```python
from build123d import *

# Parameters (mm, degrees)
ESQUISSE1_W                     = 85
ESQUISSE1_H                     = 72
BOSS_EXTRU_1_DEPTH              = 5
ESQUISSE3_R                     = 1.5
ENL_V_MAT_EXTRU_5_DEPTH         = 5
ESQUISSE5_R                     = 1.75
ENL_V_MAT_EXTRU_6_DEPTH         = 5
R_P_TITION_LIN_AIRE2_COUNT      = 6
R_P_TITION_LIN_AIRE2_PITCH      = 12
R_P_TITION_LIN_AIRE2_COUNT_DIR2 = 5
R_P_TITION_LIN_AIRE2_PITCH_DIR2 = 12
ESQUISSE6_R                     = 9.852345932
ENL_V_MAT_EXTRU_7_DEPTH         = 5
ESQUISSE8_R                     = 1.5
ENL_V_MAT_EXTRU_8_DEPTH         = 5


with BuildPart() as part:
    # Esquisse1 → Boss.-Extru.1 (new body)
    with BuildSketch(Plane.XY):
        Rectangle(ESQUISSE1_W, ESQUISSE1_H)
    extrude(amount=BOSS_EXTRU_1_DEPTH)

    # Esquisse3 → Enlèv. mat.-Extru.5 (cut)
    with BuildSketch(Plane.ZY.offset(42.5)):
        with Locations((2.5, 0)):
            Circle(ESQUISSE3_R)
    enl_v_mat_extru_5 = extrude(amount=-ENL_V_MAT_EXTRU_5_DEPTH, mode=Mode.SUBTRACT)

    # Symétrie1: Enlèv. mat.-Extru.5 across plane
    add(enl_v_mat_extru_5.mirror(Plane(origin=(0, 0, 0), x_dir=(0, 0, 1), z_dir=(1, 0, 0))), mode=Mode.SUBTRACT)

    # Esquisse5 → Enlèv. mat.-Extru.6 (cut)
    with BuildSketch(Plane.XY):
        with Locations(Location((-31.5, -25, 0), (0, 0, 180))):
            Circle(ESQUISSE5_R)
    enl_v_mat_extru_6 = extrude(amount=ENL_V_MAT_EXTRU_6_DEPTH, mode=Mode.SUBTRACT)

    # Répétition linéaire2: Enl_v. mat.-Extru.6 6 × 5
    with Locations(*[(i * R_P_TITION_LIN_AIRE2_PITCH, j * R_P_TITION_LIN_AIRE2_PITCH_DIR2, 0) for i in range(R_P_TITION_LIN_AIRE2_COUNT) for j in range(R_P_TITION_LIN_AIRE2_COUNT_DIR2) if (i, j) != (0, 0)]):
        add(enl_v_mat_extru_6, mode=Mode.SUBTRACT)

    # Esquisse6 → Enlèv. mat.-Extru.7 (cut)
    with BuildSketch(Plane.XY):
        with Locations(Location((-19.5, -13, 0), (0, 0, 180))):
            Circle(ESQUISSE6_R)
    extrude(amount=ENL_V_MAT_EXTRU_7_DEPTH, mode=Mode.SUBTRACT)

    # Esquisse8 → Enlèv. mat.-Extru.8 (cut)
    with BuildSketch(Plane(origin=(0, 36, 0), x_dir=(1, 0, 0), z_dir=(0, 1, 0))):
        with Locations(Location((0, -2.5, 0), (0, 0, 270))):
            Circle(ESQUISSE8_R)
    enl_v_mat_extru_8 = extrude(amount=-ENL_V_MAT_EXTRU_8_DEPTH, mode=Mode.SUBTRACT)

    # Symétrie2: Enlèv. mat.-Extru.8 across plane
    add(enl_v_mat_extru_8.mirror(Plane.ZX), mode=Mode.SUBTRACT)


solid = part.part
```
The listing builds one solid part. Answer for the finished solid, in the listing's coordinates (mm). A direction names the side the tool comes from. Round coordinates to 2 decimals unless told otherwise and drop trailing zeros. Write each loop counter-clockwise with the first axis right and the second up, starting at its lowest first coordinate (ties: lowest second). Pieces come first, ordered by that corner, then holes. Notation, with made-up numbers: (51.5, 83.25) -> (103.5, 83.25) arc R6 cw to (103.5, 92.25) -> close; hole circle Ø4 at (1, 85). An arc over 180 degrees is marked (long way). Use CSV: the item, a comma, the result in double quotes. Start each with the question number.
(1) Consider L1, parallel to Y at x = -19.5, z = 2.95; L2, parallel to Y at x = -7.5, z = 1.65; L3, parallel to Y at x = 38, z = 2.25. Determine where each line is inside the solid, lowest interval first. Write a range as from..to.
(2) Which of the six approach directions +Z, -Z, +X, -X, +Y, -Y give full straight-line access (tool end or side, diameter ignored) to faces 1 (the face through (-40, -0.9, 1.3)), 2 (the face through (40, -0.9, 1.3)), 3 (the face through (-19.272, -26.735, 2.465))?
(3) Section B-B on x = 16.5 is taken. Give the vertices of the cut face in (y, z).
(4) Each of these flat-tipped pins is pushed along its axis until it touches: pin 1 (3 mm diameter, centred on x = -31.5, y = -25, fed in from -Z); pin 2 (0.9 mm diameter, centred on x = 0, z = 2, fed in from +Y). Where does it stop, or does it pass through?
(5) The mould has two halves that part along Y. Classify faces 4 (the face through (-1, 1, 5)), 5 (the face through (29.79, 21.82, 2.46)), 6 (the face through (-7.272, 21.265, 2.465)), 7 (the face through (0, 31, 2)): released by +Y, released by -Y, zero draft, split by the parting line, or undercut.
(6) Section A-A on x = -19.5 is taken. Give the vertices of the cut face in (y, z).
(7) Section C-C on z = 2.5 is taken. Count the separate pieces of the cut face and the enclosed holes in it, then the cut area to 3 significant figures.
A:
1,L1,"y = -36..-26.75, -23.25..-22.85, -3.15..-2.75, 0.75..9.25, 12.75..21.25, 24.75..36"
1,L2,"y = -36..-26.75, -23.25..-14.75, -11.25..-2.75, 0.75..9.25, 12.75..21.25, 24.75..36"
1,L3,"y = -36..-1.48, 1.48..36"
2,face 1,"-X"
2,face 2,"+X"
2,face 3,"+Z, -Z"
3,outline,"(-36, 0) -> (-26.75, 0) -> (-26.75, 5) -> (-36, 5) -> close; (-23.25, 0) -> (-14.75, 0) -> (-14.75, 5) -> (-23.25, 5) -> close; (-11.25, 0) -> (-2.75, 0) -> (-2.75, 5) -> (-11.25, 5) -> close; (0.75, 0) -> (9.25, 0) -> (9.25, 5) -> (0.75, 5) -> close; (12.75, 0) -> (21.25, 0) -> (21.25, 5) -> (12.75, 5) -> close; (24.75, 0) -> (36, 0) -> (36, 5) -> (24.75, 5) -> close"
4,pin 1,"passes through"
4,pin 2,"stops at y = 31"
5,face 4,"zero draft"
5,face 5,"undercut"
5,face 6,"undercut"
5,face 7,"released by +Y"
6,outline,"(-36, 0) -> (-26.75, 0) -> (-26.75, 5) -> (-36, 5) -> close; (-23.25, 0) -> (-22.85, 0) -> (-22.85, 5) -> (-23.25, 5) -> close; (-3.15, 0) -> (-2.75, 0) -> (-2.75, 5) -> (-3.15, 5) -> close; (0.75, 0) -> (9.25, 0) -> (9.25, 5) -> (0.75, 5) -> close; (12.75, 0) -> (21.25, 0) -> (21.25, 5) -> (12.75, 5) -> close; (24.75, 0) -> (36, 0) -> (36, 5) -> (24.75, 5) -> close"
7,separate pieces,"1"
7,enclosed holes,"30"
7,area,"5,480 mm²"
